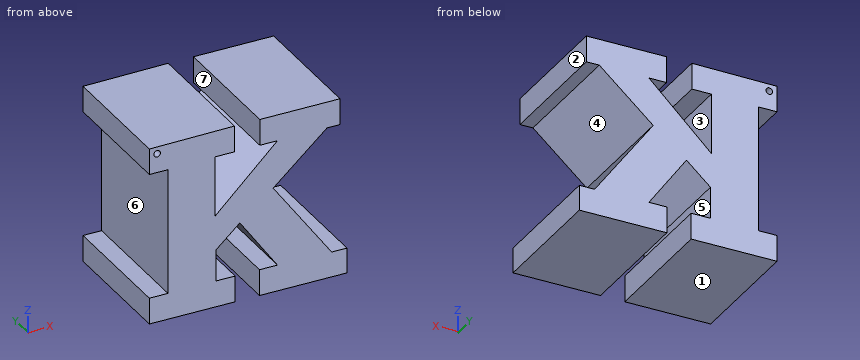
```python
from build123d import *

# Parameters (mm, degrees)
F0_R     = 0.593612
F1_DEPTH = 22.86


with BuildPart() as f1:
    # F0 (on Front) → F1 (new body)
    with BuildSketch(Plane.XZ):
        Polygon((-45.89669, 6.93236), (-61.244421, 6.752504), (-61.244421, 2.076243), (-57.887103, 2.076243), (-57.887103, -20.645589), (-61.244421, -20.645589), (-61.244421, -25.381802), (-45.776788, -25.381802), (-45.776788, -20.645589), (-49.254008, -20.645589), (-49.254008, -14.950142), (-44.937458, -11.113211), (-38.162876, -20.645589), (-41.400287, -20.645589), (-41.400287, -25.381802), (-25.632896, -25.381802), (-25.632896, -20.825444), (-28.390689, -20.825444), (-38.942251, -6.317046), (-29.230019, 2.196147), (-26.891887, 2.196147), (-26.891887, 6.93236), (-41.340336, 6.93236), (-41.340336, 2.196147), (-38.162876, 2.196147), (-49.433865, -8.715129), (-49.433865, 2.196147), (-45.89669, 2.196147), align=None)
        with Locations((-59.842687, 5.508977)):
            Circle(F0_R, mode=Mode.SUBTRACT)
    extrude(amount=F1_DEPTH)


solid = f1.part
```
Geometry: final body of the model. Coordinates: model frame, mm. Face numbers are marked on the shaded views. A direction names the side the tool comes from. Coordinates: 2 decimals unless noted, no trailing zeros. Order: outer loops, then holes, each group sorted by start corner. A loop starts at its lowest first (then second) coordinate and runs counter-clockwise, first axis right, second up. Notation, with made-up numbers: (-14, 82.25) - (5, 82.25) arc R16 ccw to (5, 89.25) - close; hole circle Ø1 at (11, 80). An arc over 180 degrees is marked (long way). Write each question's results on one line, items separated by ' | '.
1) Section B-B, the plane z = -8. Return loops of the section in (x, y), plus the area to 3 significant figures.
Results list:
outline: (-57.89, -22.86) - (-49.43, -22.86) - (-49.43, 0) - (-57.89, 0) - close; (-48.7, -22.86) - (-37.72, -22.86) - (-37.72, 0) - (-48.7, 0) - close | area: 444 mm^2
2) Pin query (flat end, axial travel): pin 1 (6.5 mm diameter, centred on y = -16, z = -18, fed in from +X); pin 2 (2.5 mm diameter, centred on x = -60, y = -11, fed in from +Z); pin 3 (8 mm diameter, centred on x = -53.5, y = -4.5, fed in from +Z); pin 4 (7 mm diameter, centred on y = -10.5, z = -8, fed in from -X). Return the tip coordinate at first contact, or that it passes through.
Results list:
pin 1: x = -25.63 | pin 2: z = 6.78 | pin 3: z = 6.89 | pin 4: x = -57.89
3) Section A-A, the plane x = -30. Return loops of the section in (y, z), plus the area to 3 significant figures.
Results list:
outline: (-22.86, -25.38) - (0, -25.38) - (0, -18.61) - (-22.86, -18.61) - close; (-22.86, 1.52) - (0, 1.52) - (0, 6.93) - (-22.86, 6.93) - close | area: 278 mm^2
4) Pull-direction query (X, two-part tool) for the marked faces 1, 2 and 3; classes: pulls with the +X half, pulls with the -X half, needs draft (parallel to the pull), parting line crosses it, or undercut.
Results list:
face 1: needs draft | face 2: pulls with the +X half | face 3: undercut
5) Section C-C, the plane x = -40. Return loops of the section in (y, z), plus the area to 3 significant figures.
Results list:
outline: (-22.86, -25.38) - (0, -25.38) - (0, -20.65) - (-22.86, -20.65) - close; (-22.86, -18.06) - (0, -18.06) - (0, 0.42) - (-22.86, 0.42) - close; (-22.86, 2.2) - (0, 2.2) - (0, 6.93) - (-22.86, 6.93) - close | area: 639 mm^2
6) Set-up query: the marked faces 4, 5, 6 and 7. Return all of +Z, -Z, +X, -X, +Y, -Y with unobstructed straight access to the full face (end or side cutting, diameter ignored); none if empty.
Results list:
face 4: +X, +Y, -Y | face 5: +Y, -Y | face 6: -X, +Y, -Y | face 7: +Z, +Y, -Y
7) Line query: line 1 (X direction, y = -5.5, z = 3.5); line 2 (X direction, y = -2.5, z = -23); line 3 (Z direction, x = -46, y = -4.25). Output: solid intervals per line, ascending. Write a range as from..to.
Results list:
line 1: -61.24..-45.9, -41.34..-26.89 | line 2: -61.24..-45.78, -41.4..-25.63 | line 3: -25.38..-20.65, -12.06..-5.39, 2.2..6.93
